Geometry check sheet. Reference: the model listing, model coordinates, mm. Face numbers are marked on the shaded views. Coordinates: 2 decimals unless noted, no trailing zeros. Loops run counter-clockwise (first coordinate to the right, second up) from the corner with the lowest first, then second, coordinate; pieces in that order, holes last. Notation, with made-up numbers: (3.5, -22) - (55.5, -22) arc R16 cw to (55.5, -9) - close; hole circle Ø10 at (75, 6.5). An arc over 180 degrees is marked (long way). One line per item, written item: value.
from build123d import *

# Parameters (mm, degrees)
SKETCH1_W           = 100
SKETCH1_H           = 28
BOSS_EXTRUDE1_DEPTH = 1
BOSS_EXTRUDE2_DEPTH = 30
BOSS_EXTRUDE3_DEPTH = 5
SKETCH4_W           = 140
SKETCH4_H           = 55
SKETCH4_W_2         = 120
SKETCH4_H_2         = 35
SKETCH4_W_3         = 110
SKETCH4_H_3         = 30
BOSS_EXTRUDE4_DEPTH = 5
SKETCH5_W           = 100
SKETCH5_H           = 28
BOSS_EXTRUDE5_DEPTH = 25
SKETCH6_R           = 2.5
CUT_EXTRUDE1_DEPTH  = 25


with BuildPart() as part:
    # Sketch1 → Boss-Extrude1 (new body)
    with BuildSketch(Plane(origin=(0, 0, 0), x_dir=(1, 0, 0), z_dir=(0, 1, 0))):
        with Locations((50, 14)):
            Rectangle(SKETCH1_W, SKETCH1_H)
    extrude(amount=BOSS_EXTRUDE1_DEPTH)



with BuildPart() as body_2:
    # Sketch2 → Boss-Extrude2 (new body)
    with BuildSketch(Plane(origin=(0, 1, 0), x_dir=(1, 0, 0), z_dir=(0, 1, 0))):
        Polygon((105, -1), (105, 14), (105, 29), (-5, 29), (-5, -1), align=None)
        Polygon((100, 28), (100, 14), (100, 0), (0, 0), (0, 28), align=None, mode=Mode.SUBTRACT)
    extrude(amount=BOSS_EXTRUDE2_DEPTH)

    # Sketch3 → Boss-Extrude3 (add)
    with BuildSketch(Plane.XZ.offset(-1)):
        Polygon((50, 3.5), (50, 1), (105, 1), (105, -29), (50, -29), (50, -31.5), (110, -31.5), (110, 3.5), align=None)
        Polygon((-5, 1), (50, 1), (50, 3.5), (-10, 3.5), (-10, -31.5), (50, -31.5), (50, -29), (-5, -29), align=None)
    extrude(amount=-BOSS_EXTRUDE3_DEPTH)

    # Sketch4 → Boss-Extrude4 (add)
    # profile 1 of 2: a face of its own
    with BuildSketch(Plane(origin=(0, 6, 0), x_dir=(1, 0, 0), z_dir=(0, 1, 0))):
        with Locations((50, 14)):
            Rectangle(SKETCH4_W, SKETCH4_H)
        with Locations((50, 14)):
            Rectangle(SKETCH4_W_2, SKETCH4_H_2, mode=Mode.SUBTRACT)
    # profile 2 of 2: a face of its own
    with BuildSketch(Plane(origin=(0, 6, 0), x_dir=(1, 0, 0), z_dir=(0, 1, 0))):
        with Locations((50, 14)):
            Rectangle(SKETCH4_W_2, SKETCH4_H_2)
        with Locations((50, 14)):
            Rectangle(SKETCH4_W_3, SKETCH4_H_3, mode=Mode.SUBTRACT)
    extrude(amount=-BOSS_EXTRUDE4_DEPTH)


with BuildPart() as part_1:
    add(part.part)

    add(body_2.part)  # Boss-Extrude5 merges body 2
    # Sketch5 → Boss-Extrude5 (add)
    with BuildSketch(Plane(origin=(0, 1, 0), x_dir=(1, 0, 0), z_dir=(0, 1, 0))):
        with Locations((50, 14)):
            Rectangle(SKETCH5_W, SKETCH5_H)
    extrude(amount=BOSS_EXTRUDE5_DEPTH)

    # Sketch6 → Cut-Extrude1 (cut)
    with BuildSketch(Plane(origin=(0, 6, 0), x_dir=(1, 0, 0), z_dir=(0, 1, 0))):
        with Locations(Location((115, 36.5, 0), (0, 0, 270))):
            Circle(SKETCH6_R)
        with Locations(Location((-15, -8.5, 0), (0, 0, 270))):
            Circle(SKETCH6_R)
    extrude(amount=-CUT_EXTRUDE1_DEPTH, mode=Mode.SUBTRACT)


solid = part_1.part
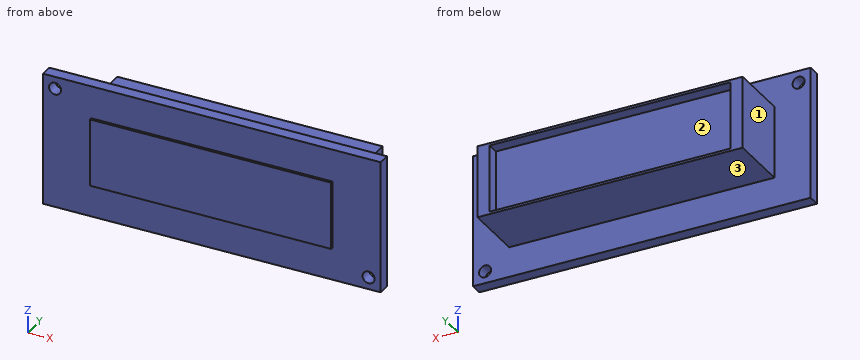
(1) Cross-section at C-C on x = 103. Record the cut outline in (y, z), and give its area (4 significant figures).
Reply:
outline: (1, -41.5) - (6, -41.5) - (6, -29) - (31, -29) - (31, 1) - (6, 1) - (6, 13.5) - (1, 13.5) - close
area: 1,025 mm2
(2) Release check for a two-part mould opening along Z. For the marked faces 1, 2 and 3 record: pulls with the +Z half, pulls with the -Z half, needs draft (parallel to the pull), parting line crosses it, or undercut.
Reply:
face 1: needs draft
face 2: undercut
face 3: pulls with the -Z half
(3) Cross-section at B-B on x = -15. Record the cut outline in (y, z).
Reply:
outline: (1, -41.5) - (6, -41.5) - (6, 6) - (1, 6) - close; (1, 11) - (6, 11) - (6, 13.5) - (1, 13.5) - close
(4) Go/stop test with flat-tipped pins: pin 1 Ø1.5 at (x, z) = (7.5, -22.5) entering from +Y; pin 2 Ø4 at (x, y) = (56, 29.5) entering from -Z; pin 3 Ø16.5 at (x, z) = (82, -2) entering from +Y; pin 4 Ø6 at (x, z) = (115, -36.5) entering from +Y. Record where each tip stops, or that it passes through.
Reply:
pin 1: y = 26
pin 2: z = -29
pin 3: y = 31
pin 4: y = 6
(5) Cross-section at A-A on z = -36.5. Record the cut outline in (x, y), and give its area (3 significant figures).
Reply:
outline: (-20, 1) - (112.5, 1) - (112.5, 6) - (-20, 6) - close; (117.5, 1) - (120, 1) - (120, 6) - (117.5, 6) - close
area: 675 mm2
(6) Material ranges on probe 1 along Z at (x, y) = (1.5, 28.5); probe 2 along X at (y, z) = (4, -36.5); probe 3 along X at (y, z) = (29, -13), recorded low to high. Write a range as from..to.
Reply:
probe 1: -29..-28, 0..1
probe 2: -20..112.5, 117.5..120
probe 3: -5..0, 100..105
(7) Cross-section at D-D on y = 28. Record the cut outline in (x, z), and give its area (3 significant figures).
Reply:
outline: (-5, -29) - (105, -29) - (105, 1) - (-5, 1) - close; hole (0, -28) - (100, -28) - (100, 0) - (0, 0) - close
area: 500 mm2
